Could you check a few things on this model? Use its own coordinates, in mm. A direction names the side the tool comes from. Coordinates: 2 decimals unless noted, no trailing zeros. Loops run counter-clockwise (first coordinate to the right, second up) from the corner with the lowest first, then second, coordinate; pieces in that order, holes last. Notation, with made-up numbers: (-33.5, -7.75) - (-18.5, -7.75) arc R28 ccw to (-18.5, 28.25) - close; hole circle Ø11 at (14, -13.75). An arc over 180 degrees is marked (long way). One line per question, with ' | ' between items. Start each with the question number.
1. I want a section at B-B, the plane y = 0. Write out the boundary of the cut face in (x, z) (3 decimals).
2. Please list where these lines run through material, in increasing order: L1, parallel to Y at x = -2.2, z = 6 (3 decimals); L2, parallel to Y at x = -1.1, z = 6 (3 decimals); L3, parallel to X at y = -1.75, z = 11.25. Write a range as [from, to].
3. We'd pull the mould along Y, two halves only. Please class faces 1 (the flat face through (-2, -8, 8)), 2 (the flat face through (-2, 9, 6)), 3 (the cylindrical face through (-2.87, 5.27, 5.92)): pulls with the +Y half, pulls with the -Y half, needs draft (parallel to the pull), parting line crosses it, or undercut.
4. I want a section at C-C, the plane x = -0.75. Write out the boundary of the cut face in (y, z) (3 decimals).
5. Which directions (+Z, -Z, +X, -X, +Y, -Y) give clear straight access to the entire face, cutting with the end or side of a thin tool? Please do faces 4 (the flat face through (-3.5, 7, 5)), 5 (the flat face through (-2, 8, 4)), 6 (the flat face through (-3.5, -7, 5)).
6. I want a section at A-A, the plane z = 3. Write out the boundary of the cut face in (x, y) (3 decimals).
7. I'm going to push flat-ended pins straight in: P1, Ø3, axis at x = -2, z = 10.5, coming from the -Y side; P2, Ø2.5, axis at y = 0, z = 3, coming from the +X side; P3, Ø1.5, axis at x = -3.5, z = 2.5, coming from the -Y side; P4, Ø1.6, axis at y = 7.75, z = 6, coming from the +X side. Where does each tip first touch, or does it pass through?
8. I want a section at D-D, the plane y = 7.75. Write out the boundary of the cut face in (x, z) (3 decimals).
from build123d import *

# Parameters (mm, degrees)
BOSS_EXTRUDE2_DEPTH  = 12
BOSS_EXTRUDE3_START  = -12
BOSS_EXTRUDE3_DEPTH  = 12
CUT_EXTRUDE6_START   = -4
CUT_EXTRUDE6_DEPTH   = 4
CUT_EXTRUDE7_REACH   = 18.348
SKETCH4_R            = 0.975
MIRROR2_START        = -4
MIRROR2_COPY_1_DEPTH = 4
CUT_EXTRUDE8_REACH   = 17.812
SKETCH6_R            = 1.025
CHAMFER1_SIZE        = 1


# Read off the part's stored shape, not the designer's step: Boss-Extrude3
with BuildPart() as part:
    # Sketch1 → Boss-Extrude2 (new body)
    with BuildSketch(Plane.XY):
        with BuildLine():
            Line((0, 6), (0, 7.5))
            ThreePointArc((0, 7.5), (-3.75510396, 6.492241081), (-6.501077384, 3.739785134))
            Line((-6.501077384, 3.739785134), (-6.501077384, -3.739785134))
            ThreePointArc((-6.501077384, -3.739785134), (-3.75510396, -6.492241081), (0, -7.5))
            Line((0, -7.5), (0, -6))
            ThreePointArc((0, -6), (-2.838133189, -5.286303056), (-5.001077384, -3.315))
            ThreePointArc((-5.001077384, -3.315), (-6, 0), (-5.001077384, 3.315))
            ThreePointArc((-5.001077384, 3.315), (-2.838133189, 5.286303056), (0, 6))
        make_face()
        with BuildLine():
            Line((-5.001077384, -3.315), (-5.001077384, 3.315))
            ThreePointArc((-5.001077384, 3.315), (-6, 0), (-5.001077384, -3.315))
        make_face()
    extrude(amount=BOSS_EXTRUDE2_DEPTH)

    # Boss-Extrude3 outline → Boss-Extrude3 (add)
    with BuildSketch(Plane.XY.offset(12).offset(BOSS_EXTRUDE3_START)):
        with BuildLine():
            ThreePointArc((-3.5, 6.633249581), (-1.802862744, 7.280088319), (0, 7.5))
            Line((0, 7.5), (0, 9))
            Line((0, 9), (-3.5, 9))
            Line((-3.5, 9), (-3.5, 6.633249581))
        make_face()
    boss_extrude3 = extrude(amount=BOSS_EXTRUDE3_DEPTH)

    # Sketch3 → Cut-Extrude6 (cut)
    with BuildSketch(Plane.XY.offset(12).offset(CUT_EXTRUDE6_START)):
        with BuildLine():
            Line((-4.617876388, 10.846765639), (-4.617876388, 5.909756142))
            ThreePointArc((-4.617876388, 5.909756142), (-1.858071818, 7.266193578), (1.214101671, 7.401078106))
            Line((1.214101671, 7.401078106), (1.214101671, 10.846765639))
            Line((1.214101671, 10.846765639), (-4.617876388, 10.846765639))
        make_face()
    cut_extrude6 = extrude(amount=CUT_EXTRUDE6_DEPTH, mode=Mode.SUBTRACT)

    # Mirror1: Cut-Extrude6 across plane
    add(cut_extrude6.mirror(Plane.XY.offset(6)), mode=Mode.SUBTRACT)

    # Sketch4 → Cut-Extrude7 (cut, up to next)
    with BuildSketch(Plane(origin=(0, 0, 0), x_dir=(0, 0, -1), z_dir=(1, 0, 0)), mode=Mode.PRIVATE) as cut_extrude7_sk1:
        with Locations((-6, 7.75)):
            Circle(SKETCH4_R)
    cut_extrude7_tool1 = extrude(cut_extrude7_sk1.sketch, amount=-CUT_EXTRUDE7_REACH, mode=Mode.PRIVATE) & part.part
    cut_extrude7 = cut_extrude7_tool1.solids().sort_by_distance((0, 7.75, 6))[0]
    add(cut_extrude7, mode=Mode.SUBTRACT)

    # Mirror2: Boss-Extrude3, Cut-Extrude6, Cut-Extrude7 across plane
    add(boss_extrude3.mirror(Plane.ZX))
    add(cut_extrude6.mirror(Plane.ZX), mode=Mode.SUBTRACT)
    add(cut_extrude7.mirror(Plane.ZX), mode=Mode.SUBTRACT)

    # Mirror2 copy 1 sketch → Mirror2 copy 1 (cut)
    with BuildSketch(Plane(origin=(0, 0, 0), x_dir=(1, 0, 0), z_dir=(0, 0, -1)).offset(MIRROR2_START)):
        with BuildLine():
            Line((-4.617876388, 10.846765639), (-4.617876388, 5.909756142))
            ThreePointArc((-4.617876388, 5.909756142), (-1.858071818, 7.266193578), (1.214101671, 7.401078106))
            Line((1.214101671, 7.401078106), (1.214101671, 10.846765639))
            Line((1.214101671, 10.846765639), (-4.617876388, 10.846765639))
        make_face()
    extrude(amount=MIRROR2_COPY_1_DEPTH, mode=Mode.SUBTRACT)

    # Sketch6 → Cut-Extrude8 (cut, up to next)
    with BuildSketch(Plane(origin=(-5.001077384, 0, 0), x_dir=(0, 0, -1), z_dir=(1, 0, 0)), mode=Mode.PRIVATE) as cut_extrude8_sk1:
        with Locations((-9, 0)):
            Circle(SKETCH6_R)
    cut_extrude8_tool1 = extrude(cut_extrude8_sk1.sketch, amount=-CUT_EXTRUDE8_REACH, mode=Mode.PRIVATE) & part.part
    # Sketch6 → Cut-Extrude8 (cut, up to next)
    with BuildSketch(Plane(origin=(-5.001077384, 0, 0), x_dir=(0, 0, -1), z_dir=(1, 0, 0)), mode=Mode.PRIVATE) as cut_extrude8_sk2:
        with Locations((-3, 0)):
            Circle(SKETCH6_R)
    cut_extrude8_tool2 = extrude(cut_extrude8_sk2.sketch, amount=-CUT_EXTRUDE8_REACH, mode=Mode.PRIVATE) & part.part
    add(cut_extrude8_tool1.solids().sort_by_distance((-5.001077, 0, 9))[0], mode=Mode.SUBTRACT)
    add(cut_extrude8_tool2.solids().sort_by_distance((-5.001077, 0, 3))[0], mode=Mode.SUBTRACT)

    # Chamfer1
    chamfer1_edges = [part.edges().sort_by_distance(p)[0] for p in [
        (-5.001077384, 0, 10.025),
        (-5.001077384, 0, 4.025),
    ]]
    chamfer(chamfer1_edges, length=CHAMFER1_SIZE)


solid = part.part
Results are:
1) outline: (-6.501, 0) - (-5.001, 0) - (-5.001, 0.975) - (-6.001, 1.975) - (-6.501, 1.975) - close; (-6.501, 4.025) - (-6.001, 4.025) - (-5.001, 5.025) - (-5.001, 6.975) - (-6.001, 7.975) - (-6.501, 7.975) - close; (-6.501, 10.025) - (-6.001, 10.025) - (-5.001, 11.025) - (-5.001, 12) - (-6.501, 12) - close
2) L1: y = [-9, -8.725], [-6.775, -5.582], [5.582, 6.775], [8.725, 9] | L2: y = [-9, -8.725], [-6.775, -5.898], [5.898, 6.775], [8.725, 9] | L3: x = [-6.5, -5]
3) face 1: needs draft | face 2: pulls with the +Y half | face 3: undercut
4) outline: (-9, 4) - (-7.462, 4) - (-7.462, 0) - (-5.953, 0) - (-5.953, 12) - (-7.462, 12) - (-7.462, 8) - (-9, 8) - close; (5.953, 0) - (7.462, 0) - (7.462, 4) - (9, 4) - (9, 8) - (7.462, 8) - (7.462, 12) - (5.953, 12) - close; hole circle Ø1.95 at (-7.75, 6); hole circle Ø1.95 at (7.75, 6)
5) face 4: +Z, -Z, -X, +Y | face 5: -Z, -X, +Y | face 6: +Z, -Z, -X, -Y
6) outline: (-6.501, -3.74) arc R7.5 ccw to (0, -7.5) - (0, -6) arc R6 cw to (-5.001, -3.315) - (-5.001, -2.025) - (-6.001, -1.025) - (-6.501, -1.025) - close; (-6.501, 1.025) - (-6.001, 1.025) - (-5.001, 2.025) - (-5.001, 3.315) arc R6 cw to (0, 6) - (0, 7.5) arc R7.5 ccw to (-6.501, 3.74) - close
7) P1: stops at y = -7.48 | P2: stops at x = -5.78 | P3: stops at y = -6.98 | P4: passes through
8) outline: (-3.5, 4) - (0, 4) - (0, 5.025) - (-3.5, 5.025) - close; (-3.5, 6.975) - (0, 6.975) - (0, 8) - (-3.5, 8) - close
